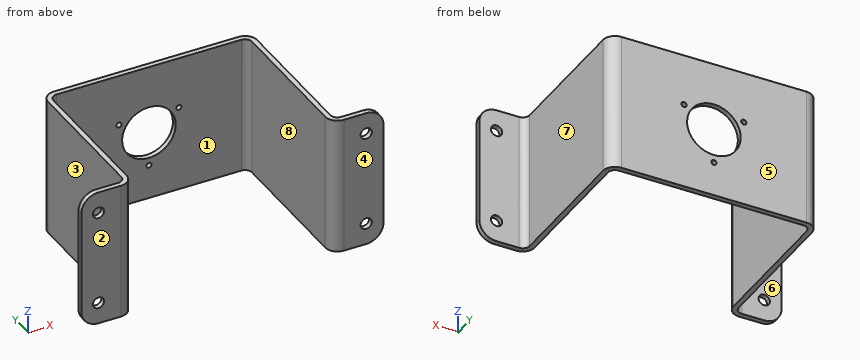
```python
from build123d import *

# Parameters (mm, degrees)
TABAN_FLAN_1_DEPTH    = 80
IZIM2_R               = 1.5
KES_EKSTR_ZYON1_DEPTH = 10
IZIM3_R               = 15.5
KES_EKSTR_ZYON2_DEPTH = 10
RADYUS1_R             = 10
IZIM4_R               = 3.25
KES_EKSTR_ZYON3_DEPTH = 10


# Read off the part's stored shape, not the designer's step: Taban-Flanş1
with BuildPart() as part:
    # Taban-Flanş1 outline → Taban-Flanş1 (new body)
    with BuildSketch(Plane.XY):
        with BuildLine():
            Line((152, 0), (175, 0))
            Line((175, 0), (175, 3))
            Line((175, 3), (152, 3))
            ThreePointArc((152, 3), (149.171572875, 4.171572875), (148, 7))
            Line((148, 7), (148, 86))
            ThreePointArc((148, 86), (145.949747468, 90.949747468), (141, 93))
            Line((141, 93), (34, 93))
            ThreePointArc((34, 93), (29.050252532, 90.949747468), (27, 86))
            Line((27, 86), (27, 7))
            ThreePointArc((27, 7), (25.828427125, 4.171572875), (23, 3))
            Line((23, 3), (0, 3))
            Line((0, 3), (0, 0))
            Line((0, 0), (23, 0))
            ThreePointArc((23, 0), (27.949747468, 2.050252532), (30, 7))
            Line((30, 7), (30, 86))
            ThreePointArc((30, 86), (31.171572875, 88.828427125), (34, 90))
            Line((34, 90), (141, 90))
            ThreePointArc((141, 90), (143.828427125, 88.828427125), (145, 86))
            Line((145, 86), (145, 7))
            ThreePointArc((145, 7), (147.050252532, 2.050252532), (152, 0))
        make_face()
    extrude(amount=TABAN_FLAN_1_DEPTH)

    # Çizim2 → Kes-Ekstrüzyon1 (cut)
    with BuildSketch(Plane(origin=(0, 93, 0), x_dir=(1, 0, 0), z_dir=(0, 1, 0))):
        with Locations(Location((87.5, -20, 0), (0, 0, 270))):
            Circle(IZIM2_R)
        with Locations(Location((104.820508076, -50, 0), (0, 0, 270))):
            Circle(IZIM2_R)
        with Locations(Location((70.179491924, -50, 0), (0, 0, 270))):
            Circle(IZIM2_R)
    extrude(amount=-KES_EKSTR_ZYON1_DEPTH, mode=Mode.SUBTRACT)

    # Çizim3 → Kes-Ekstrüzyon2 (cut)
    with BuildSketch(Plane(origin=(0, 93, 0), x_dir=(1, 0, 0), z_dir=(0, 1, 0))):
        with Locations(Location((87.5, -40, 0), (0, 0, 270))):
            Circle(IZIM3_R)
    extrude(amount=-KES_EKSTR_ZYON2_DEPTH, mode=Mode.SUBTRACT)

    # Radyus1
    radyus1_edges = [part.edges().sort_by_distance(p)[0] for p in [
        (0, 1.5, 0),
        (175, 1.5, 0),
        (0, 1.5, 80),
        (175, 1.5, 80),
    ]]
    fillet(radyus1_edges, radius=RADYUS1_R)

    # Çizim4 → Kes-Ekstrüzyon3 (cut)
    with BuildSketch(Plane(origin=(0, 3, 0), x_dir=(1, 0, 0), z_dir=(0, 1, 0))):
        with Locations(Location((10, -12.5, 0), (0, 0, 270))):
            Circle(IZIM4_R)
        with Locations(Location((10, -67.5, 0), (0, 0, 270))):
            Circle(IZIM4_R)
        with Locations(Location((165, -67.5, 0), (0, 0, 270))):
            Circle(IZIM4_R)
        with Locations(Location((165, -12.5, 0), (0, 0, 270))):
            Circle(IZIM4_R)
    extrude(amount=-KES_EKSTR_ZYON3_DEPTH, mode=Mode.SUBTRACT)


solid = part.part
```
Could you check a few things on this model? Use its own coordinates, in mm. Face numbers are marked on the shaded views. A direction names the side the tool comes from. Coordinates: 2 decimals unless noted, no trailing zeros. Order: outer loops, then holes, each group sorted by start corner. A loop starts at its lowest first (then second) coordinate and runs counter-clockwise, first axis right, second up. Notation, with made-up numbers: M 19,-20 L 33,-20 A15 cw 33,-14 Z; hole C -13.75,-11.5 d3. An arc over 180 degrees is marked long. Use a Markdown table: item, result. Add a question column.
Q1. I'm going to push flat-ended pins straight in: pin 1 (23.5 mm diameter, centred on y = 43, z = 33.5, fed in from -X); pin 2 (12 mm diameter, centred on y = 15, z = 35.5, fed in from +X); pin 3 (4 mm diameter, centred on x = 87.5, z = 20, fed in from -Y). Where does each tip first touch, or does it pass through?
Q2. I want a section at B-B on z = 67.5. List the corners of the cut face in (x, y) for me.
Q3. I want a section at C-C on z = 29. List the corners of the cut face in (x, y) for me.
Q4. Which directions (+Z, -Z, +X, -X, +Y, -Y) give clear straight access to the entire face, cutting with the end or side of a thin tool? Please do the marked faces 4, 5, 6, 7 and 8.
Q5. I want a section at D-D on x = 84. List the corners of the cut face in (y, z) for me, then the cut area to 3 significant figures.
Q6. We'd pull the mould along X, two halves only. Please class the marked faces 1, 2 and 3: pulls with the +X half, pulls with the -X half, needs draft (parallel to the pull), parting line crosses it, or undercut.
Q7. If I drill on L1, parallel to Z at x = 165, y = 2.2; L2, parallel to X at y = 83, z = 37.5; L3, parallel to X at y = 1.6, z = 12.5, over which ranges is the centre line in solid material (lowest first)?
Q8. I want a section at A-A on y = 59. List the corners of the cut face in (x, z) for me, then the cut area to 3 significant figures.
Checked values:
| question | item | result |
|---|---|---|
| 1 | pin 1 | x = 27 |
| 1 | pin 2 | x = 148 |
| 1 | pin 3 | y = 90 |
| 2 | outline | M 0,0 L 6.75,0 L 6.75,3 L 0,3 Z; M 13.25,0 L 23,0 A7 ccw 30,7 L 30,86 A4 cw 34,90 L 141,90 A4 cw 145,86 L 145,7 A7 ccw 152,0 L 161.75,0 L 161.75,3 L 152,3 A4 cw 148,7 L 148,86 A7 ccw 141,93 L 34,93 A7 ccw 27,86 L 27,7 A4 cw 23,3 L 13.25,3 Z; M 168.25,0 L 175,0 L 175,3 L 168.25,3 Z |
| 3 | outline | M 0,0 L 23,0 A7 ccw 30,7 L 30,86 A4 cw 34,90 L 76.58,90 L 76.58,93 L 34,93 A7 ccw 27,86 L 27,7 A4 cw 23,3 L 0,3 Z; M 98.42,90 L 141,90 A4 cw 145,86 L 145,7 A7 ccw 152,0 L 175,0 L 175,3 L 152,3 A4 cw 148,7 L 148,86 A7 ccw 141,93 L 98.42,93 Z |
| 4 | face 4 | +Z, -Z, +X, -X, -Y |
| 4 | face 5 | +Z, -Z, +X, -X, +Y |
| 4 | face 6 | +Z, -Z, -X, +Y |
| 4 | face 7 | +Z, -Z, +X, +Y |
| 4 | face 8 | +Z, -Z, -Y |
| 5 | outline | M 90,0 L 93,0 L 93,24.9 L 90,24.9 Z; M 90,55.1 L 93,55.1 L 93,80 L 90,80 Z |
| 5 | area | 149 mm² |
| 6 | face 1 | undercut |
| 6 | face 2 | needs draft |
| 6 | face 3 | pulls with the -X half |
| 7 | L1 | 0 to 9.25, 15.75 to 64.25, 70.75 to 80 |
| 7 | L2 | 27 to 30, 145 to 148 |
| 7 | L3 | 0 to 6.75, 13.25 to 27.45, 147.55 to 161.75, 168.25 to 175 |
| 8 | outline | M 27,0 L 30,0 L 30,80 L 27,80 Z; M 145,0 L 148,0 L 148,80 L 145,80 Z |
| 8 | area | 480 mm² |
